The listing builds one solid part. Answer for the finished solid, in the listing's coordinates (mm). A direction names the side the tool comes from. Give positions to 0.01 mm unless a question says otherwise; leave off trailing zeros. Order: outer loops, then holes, each group sorted by start corner. A loop starts at its lowest first (then second) coordinate and runs counter-clockwise, first axis right, second up. Notation, with made-up numbers: (-31.5, -12) - (15.5, -12) arc R30 ccw to (15.5, 17) - close; hole circle Ø8 at (10.5, 56). An arc over 180 degrees is marked (long way). Answer as CSV lines item,"result". Start each with the question number.
1. Section C-C on y = 32.5 is taken. Give the vertices of the cut face in (x, z), and give its area (3 significant figures).
2. Consider line 1 along Y through (x, z) = (-8, -44); line 2 along Y through (x, z) = (-8.85, -28.5); line 3 along Y through (x, z) = (-16, -11). Determine where each line is inside the solid, lowest interval first. Write a range as [from, to].
3. Section A-A on z = -13 is taken. Give the vertices of the cut face in (x, y).
4. Section B-B on x = -2 is taken. Give the vertices of the cut face in (y, z), and give its area (3 significant figures).
5. Determine the mould class of faces 1 (the flat face through (-6, 61, -33.5)), 2 (the flat face through (-28.254, -1.375, -26.087)), 3 (the flat face through (-13, 1, 3)), 4 (the flat face through (2.254, -1.375, -26.087)) for opening direction X: +X half, -X half, draft (parallel to the pull), parting line (faces both ways), or undercut.
6. Section D-D on y = 17 is taken. Give the vertices of the cut face in (x, z), and give its area (3 significant figures).
7. Flat-ended cylindrical pins translate along their axes: pin 1 (6 mm diameter, centred on x = -9.5, z = -23.5, fed in from -Y); pin 2 (23 mm diameter, centred on y = 31, z = -32.5, fed in from -X); pin 3 (3 mm diameter, centred on x = -14.5, z = -25, fed in from -Y); pin 4 (12 mm diameter, centred on x = -22, y = 42.5, fed in from +Z). Find the tip coordinate at first contact, or state that the pin passes through.
8. Which of the six approach directions +Z, -Z, +X, -X, +Y, -Y give full straight-line access (tool end or side, diameter ignored) to faces 5 (the flat face through (4, 58, -31)), 6 (the flat face through (-6, 41, -50)), 7 (the cylindrical face through (-7.958, 17.526, -45.669)), 8 (the flat face through (-26, -2, -26))?
from build123d import *

# Parameters (mm, degrees)
SKETCH1_W           = 26
SKETCH1_H           = 53
SKETCH1_W_2         = 20
SKETCH1_H_2         = 10
BOSS_EXTRUDE1_DEPTH = 5
SKETCH2_W           = 31
SKETCH2_H           = 59
SKETCH2_W_2         = 26
SKETCH2_H_2         = 53
BOSS_EXTRUDE2_DEPTH = 10
SKETCH3_W           = 31
SKETCH3_H           = 59
BOSS_EXTRUDE3_DEPTH = 3
SKETCH4_W           = 6
SKETCH4_H           = 46
BOSS_EXTRUDE4_DEPTH = 55
SKETCH5_R           = 1.75
SKETCH5_R_2         = 13.5
CUT_EXTRUDE1_DEPTH  = 24.5
CHAMFER1_SIZE       = 0.5
CHAMFER1_SIZE2      = 7.150333128
SKETCH6_W           = 46
SKETCH6_H           = 7
BOSS_EXTRUDE5_DEPTH = 14
SKETCH7_W           = 5
SKETCH7_H           = 5
CUT_EXTRUDE2_DEPTH  = 5


with BuildPart() as part:
    # Sketch1 → Boss-Extrude1 (new body)
    with BuildSketch(Plane(origin=(0, 0, 0), x_dir=(1, 0, 0), z_dir=(0, 1, 0))):
        with Locations((-13, 26.5)):
            Rectangle(SKETCH1_W, SKETCH1_H)
        with Locations((-13, 27)):
            Rectangle(SKETCH1_W_2, SKETCH1_H_2, mode=Mode.SUBTRACT)
        with Locations((-13, 43)):
            Rectangle(SKETCH1_W_2, SKETCH1_H_2, mode=Mode.SUBTRACT)
        with Locations((-13, 11)):
            Rectangle(SKETCH1_W_2, SKETCH1_H_2, mode=Mode.SUBTRACT)
    extrude(amount=BOSS_EXTRUDE1_DEPTH)

    # Sketch2 → Boss-Extrude2 (add)
    with BuildSketch(Plane(origin=(0, 5, 0), x_dir=(1, 0, 0), z_dir=(0, 1, 0))):
        with Locations((-13, 26.5)):
            Rectangle(SKETCH2_W, SKETCH2_H)
        with Locations((-13, 26.5)):
            Rectangle(SKETCH2_W_2, SKETCH2_H_2, mode=Mode.SUBTRACT)
    extrude(amount=-BOSS_EXTRUDE2_DEPTH)

    # Sketch3 → Boss-Extrude3 (add)
    with BuildSketch(Plane(origin=(0, 5, 0), x_dir=(1, 0, 0), z_dir=(0, 1, 0))):
        with Locations((-13, 26.5)):
            Rectangle(SKETCH3_W, SKETCH3_H)
    extrude(amount=BOSS_EXTRUDE3_DEPTH)

    # Sketch4 → Boss-Extrude4 (add)
    with BuildSketch(Plane(origin=(0, 8, 0), x_dir=(1, 0, 0), z_dir=(0, 1, 0))):
        with Locations((-8, 27)):
            Rectangle(SKETCH4_W, SKETCH4_H)
    extrude(amount=BOSS_EXTRUDE4_DEPTH)

    # Sketch5 → Cut-Extrude1 (cut, through all)
    with BuildSketch(Plane(origin=(-5, 0, 0), x_dir=(0, 0, -1), z_dir=(1, 0, 0))):
        with Locations((44, 17)):
            Circle(SKETCH5_R)
        with Locations((13, 17)):
            Circle(SKETCH5_R)
        with Locations((13, 48)):
            Circle(SKETCH5_R)
        with Locations((44, 48)):
            Circle(SKETCH5_R)
        with Locations((28.5, 32.5)):
            Circle(SKETCH5_R_2)
    extrude(amount=-CUT_EXTRUDE1_DEPTH, mode=Mode.SUBTRACT)

    # Chamfer1
    chamfer1_edges = [part.edges().sort_by_distance(p)[0] for p in [
        (-28.5, -5, -26.5),
        (2.5, -5, -26.5),
    ]]
    chamfer1_side = [part.faces().sort_by_distance(p)[0] for p in [
        (-13, -5, -55.333516692),
    ]]
    chamfer(chamfer1_edges, length=CHAMFER1_SIZE, length2=CHAMFER1_SIZE2, reference=chamfer1_side[0])

    # Sketch6 → Boss-Extrude5 (add)
    with BuildSketch(Plane(origin=(-5, 0, 0), x_dir=(0, 0, -1), z_dir=(1, 0, 0))):
        with Locations((27, 59.5)):
            Rectangle(SKETCH6_W, SKETCH6_H)
    extrude(amount=BOSS_EXTRUDE5_DEPTH)

    # Sketch7 → Cut-Extrude2 (cut)
    with BuildSketch(Plane(origin=(0, 63, 0), x_dir=(1, 0, 0), z_dir=(0, 1, 0))):
        with Locations((-6, 31)):
            Rectangle(SKETCH7_W, SKETCH7_H)
        with Locations((4, 31)):
            Rectangle(SKETCH7_W, SKETCH7_H)
        with Locations((-6, 8)):
            Rectangle(SKETCH7_W, SKETCH7_H)
        with Locations((4, 8)):
            Rectangle(SKETCH7_W, SKETCH7_H)
    extrude(amount=-CUT_EXTRUDE2_DEPTH, mode=Mode.SUBTRACT)


solid = part.part
Checks:
1,outline,"(-11, -50) - (-5, -50) - (-5, -42) - (-11, -42) - close; (-11, -15) - (-5, -15) - (-5, -4) - (-11, -4) - close"
1,area,"114 mm²"
2,line 1,"y = [5, 15.25], [18.75, 46.25], [49.75, 63]"
2,line 2,"y = [5, 19], [46, 63]"
2,line 3,"y = [5, 8]"
3,outline,"(-28.5, 2.15) - (-28, -5) - (-26, -5) - (-26, 0) - (-23, 0) - (-23, 5) - (-3, 5) - (-3, 0) - (0, 0) - (0, -5) - (2, -5) - (2.5, 2.15) - (2.5, 8) - (-5, 8) - (-5, 15.25) - (-11, 15.25) - (-11, 8) - (-28.5, 8) - close; (-11, 18.75) - (-5, 18.75) - (-5, 46.25) - (-11, 46.25) - close; (-11, 49.75) - (-5, 49.75) - (-5, 56) - (9, 56) - (9, 63) - (-11, 63) - close"
4,outline,"(-5, -56) - (8, -56) - (8, 3) - (-5, 3) - (-5, 0) - (0, 0) - (0, -53) - (-5, -53) - close; (56, -50) - (63, -50) - (63, -4) - (56, -4) - close"
4,area,"824 mm²"
5,face 1,"undercut"
5,face 2,"-X half"
5,face 3,"draft"
5,face 4,"+X half"
6,outline,"(-11, -50) - (-5, -50) - (-5, -45.75) - (-11, -45.75) - close; (-11, -42.25) - (-5, -42.25) - (-5, -14.75) - (-11, -14.75) - close; (-11, -11.25) - (-5, -11.25) - (-5, -4) - (-11, -4) - close"
6,area,"234 mm²"
7,pin 1,"stops at y = 0"
7,pin 2,"stops at x = -11"
7,pin 3,"stops at y = 5"
7,pin 4,"passes through"
8,face 5,"+Y"
8,face 6,"-Z, +X, -X, +Y"
8,face 7,"+X, -X"
8,face 8,"-Y"
